Input: part model. Units: mm. Frame: model coordinates. Face numbers are marked on the shaded views. A direction names the side the tool comes from. Coordinates: 2 decimals unless noted, no trailing zeros. Loops run counter-clockwise (first coordinate to the right, second up) from the corner with the lowest first, then second, coordinate; pieces in that order, holes last. Notation, with made-up numbers: (58, 87.25) - (99, 87.25) arc R29 ccw to (99, 123.25) - close; hole circle Ø5 at (74, 24). An arc over 180 degrees is marked (long way). Write item = value, one per line. Start each with the question number.
from build123d import *

# Parameters (mm, degrees)
SKETCH_1_W          = 60
SKETCH_1_H          = 30
EXTRUDE_1_DEPTH     = 9
SKETCH_2_W          = 25
SKETCH_2_H          = 55
EXTRUDE_2_DEPTH     = 10
SKETCH_3_W          = 20
SKETCH_3_H          = 40
EXTRUDE_3_DEPTH     = 25
SKETCH_4_W          = 20
SKETCH_4_H          = 5
EXTRUDE_4_DEPTH     = 4
FILLET_1_R          = 4
FILLET_2_R          = 3
FILLET_3_R          = 3
EXTRUDE_5_DEPTH     = 4
EXTRUDE_6_DEPTH     = 4
FILLET_4_R          = 2
CHAMFER_1_SIZE      = 1
SKETCH_7_W          = 40
SKETCH_7_H          = 20
EXTRUDE_7_DEPTH     = 25
SKETCH_8_W          = 5
SKETCH_8_H          = 20
EXTRUDE_8_DEPTH     = 4
CHAMFER_2_SIZE      = 1
FILLET_6_R          = 2
SKETCH_9_R          = 3
CUT_EXTRUDE_1_DEPTH = 2


with BuildPart() as part:
    # 草图1 → 凸台-拉伸1 (new body)
    with BuildSketch(Plane.XY):
        Rectangle(SKETCH_1_W, SKETCH_1_H)
    extrude(amount=EXTRUDE_1_DEPTH)

    # 草图2 → 凸台-拉伸2 (add)
    with BuildSketch(Plane.XZ.offset(15)):
        with Locations((42.5, -3.5)):
            Rectangle(SKETCH_2_W, SKETCH_2_H)
    extrude(amount=-EXTRUDE_2_DEPTH)

    # 草图3 → 凸台-拉伸3 (add)
    with BuildSketch(Plane(origin=(0, -5, 0), x_dir=(1, 0, 0), z_dir=(0, 1, 0))):
        with Locations((42.5, 3.5)):
            Rectangle(SKETCH_3_W, SKETCH_3_H)
    extrude(amount=EXTRUDE_3_DEPTH)

    # 草图4 → 凸台-拉伸4 (add)
    with BuildSketch(Plane(origin=(0, -5, 0), x_dir=(1, 0, 0), z_dir=(0, 1, 0))):
        with Locations((42.5, 26)):
            Rectangle(SKETCH_4_W, SKETCH_4_H)
        with Locations((42.5, -19)):
            Rectangle(SKETCH_4_W, SKETCH_4_H)
    extrude(amount=EXTRUDE_4_DEPTH)

    # 圆角1
    fillet_1_edges = [part.edges().sort_by_distance(p)[0] for p in [
        (30, -10, -31),
        (30, -10, 24),
        (55, -10, 24),
        (55, -10, -31),
    ]]
    fillet(fillet_1_edges, radius=FILLET_1_R)

    # 圆角2
    fillet_2_edges = [part.edges().sort_by_distance(p)[0] for p in [
        (52.5, -3, -28.5),
        (32.5, -3, -28.5),
        (52.5, -3, 21.5),
        (32.5, -3, 21.5),
    ]]
    fillet(fillet_2_edges, radius=FILLET_2_R)

    # 圆角3
    fillet_3_edges = [part.edges().sort_by_distance(p)[0] for p in [
        (-30, -15, 4.5),
        (-30, 15, 4.5),
        (30, 15, 4.5),
    ]]
    fillet(fillet_3_edges, radius=FILLET_3_R)

    # 草图5 → 凸台-拉伸5 (add)
    with BuildSketch(Plane.XZ.offset(15)):
        with BuildLine():
            Line((34, 24), (66, 24))
            ThreePointArc((66, 24), (70, 20), (66, 16))
            Line((66, 16), (34, 16))
            ThreePointArc((34, 16), (30, 20), (34, 24))
        make_face()
        with BuildLine():
            Line((35, 10), (75, 10))
            ThreePointArc((75, 10), (80, 5), (75, 0))
            Line((75, 0), (35, 0))
            ThreePointArc((35, 0), (30, 5), (35, 10))
        make_face()
    extrude_5 = extrude(amount=EXTRUDE_5_DEPTH)

    # 镜向1: 凸台-拉伸5 across plane
    add(extrude_5.mirror(Plane(origin=(0, 0, -3.5), x_dir=(1, 0, 0), z_dir=(0, 0, -1))))

    # 草图6 → 凸台-拉伸6 (add)
    with BuildSketch(Plane(origin=(0, -15, 0), x_dir=(1, 0, 0), z_dir=(0, 1, 0))):
        Polygon((62, 34), (77, 6), (127, 6), (127, 10.5), align=None)
    extrude_6 = extrude(amount=EXTRUDE_6_DEPTH)

    # 镜向2: 凸台-拉伸6 across plane
    add(extrude_6.mirror(Plane(origin=(0, 0, -3.5), x_dir=(1, 0, 0), z_dir=(0, 0, -1))))

    # 圆角4
    # the kernel refuses this fillet: 2 mm, written as the material it takes off along each edge
    with BuildSketch(Plane(origin=(62, -15, -34), x_dir=(0.47222141251542, 0, 0.8814799700287814), z_dir=(0, 1, 0))) as fillet_4_piece_1:
        with BuildLine():
            CenterArc((FILLET_4_R * 2.60886248276, FILLET_4_R), FILLET_4_R, 131.944537695, 138.055462305)
            Line((FILLET_4_R * 1.94045155385, FILLET_4_R * 1.74379219551), (0, 0))
            Line((0, 0), (FILLET_4_R * 2.60886248276, 0))
        make_face()
    extrude(amount=17.044312414, mode=Mode.SUBTRACT)
    with BuildSketch(Plane(origin=(62, -15, 27), x_dir=(0.47222141251541977, 0, -0.8814799700287816), z_dir=(0, 1, 0))) as fillet_4_piece_2:
        with BuildLine():
            CenterArc((FILLET_4_R * 2.60886248276, -FILLET_4_R), FILLET_4_R, 90, 138.055462305)
            Line((FILLET_4_R * 1.94045155385, -FILLET_4_R * 1.74379219551), (0, 0))
            Line((0, 0), (FILLET_4_R * 2.60886248276, 0))
        make_face()
    extrude(amount=17.044312414, mode=Mode.SUBTRACT)

    # 倒角1
    chamfer_1_edges = [part.edges().sort_by_distance(p)[0] for p in [
        (32.5, 20, -3.5),
        (42.5, 20, 16.5),
        (52.5, 20, -3.5),
        (42.5, 20, -23.5),
    ]]
    chamfer(chamfer_1_edges, length=CHAMFER_1_SIZE)

    # 草图7 → 凸台-拉伸7 (add)
    with BuildSketch(Plane(origin=(0, 0, 0), x_dir=(-1, 0, 0), z_dir=(0, 0, -1))):
        Rectangle(SKETCH_7_W, SKETCH_7_H)
    extrude(amount=EXTRUDE_7_DEPTH)

    # 草图8 → 凸台-拉伸8 (add)
    with BuildSketch(Plane(origin=(0, 0, 0), x_dir=(-1, 0, 0), z_dir=(0, 0, -1))):
        with Locations((22.5, 0)):
            Rectangle(SKETCH_8_W, SKETCH_8_H)
        with Locations((-22.5, 0)):
            Rectangle(SKETCH_8_W, SKETCH_8_H)
    extrude(amount=EXTRUDE_8_DEPTH)

    # 倒角2
    chamfer_2_edges = [part.edges().sort_by_distance(p)[0] for p in [
        (-20, 0, -25),
        (0, 10, -25),
        (20, 0, -25),
        (0, -10, -25),
    ]]
    chamfer(chamfer_2_edges, length=CHAMFER_2_SIZE)

    # 圆角6
    fillet_6_edges = [part.edges().sort_by_distance(p)[0] for p in [
        (-25, -10, -2),
        (-25, 10, -2),
        (25, 10, -2),
        (25, -10, -2),
    ]]
    fillet(fillet_6_edges, radius=FILLET_6_R)

    # 草图9 → 切除-拉伸1 (cut)
    with BuildSketch(Plane.XY.offset(9)):
        with Locations((-10, 0)):
            Circle(SKETCH_9_R)
    extrude(amount=-CUT_EXTRUDE_1_DEPTH, mode=Mode.SUBTRACT)


solid = part.part
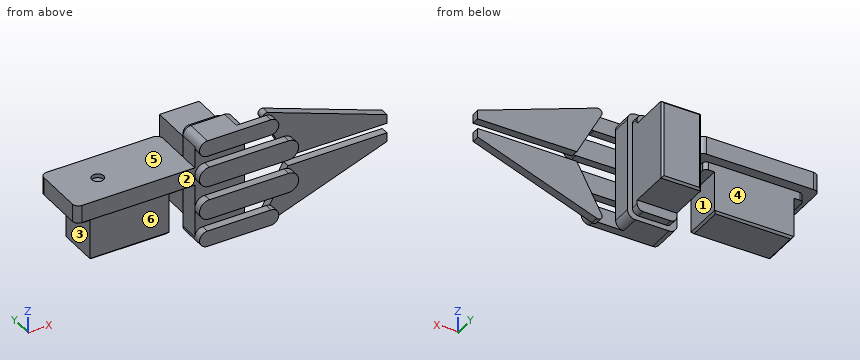
Item 1: Cut plane B-B on z = -20. Return loops of the section in (x, y).
Item 2: Pull-direction query (X, two-part tool) for the marked faces 1, 2 and 3; classes: pulls with the +X half, pulls with the -X half, needs draft (parallel to the pull), parting line crosses it, or undercut.
Item 3: Cut plane C-C on x = 98. Return loops of the section in (y, z).
Item 4: Ray query, line 1 (Z direction, x = 65.5, y = -16); line 2 (Y direction, x = -10, z = 7.7); line 3 (X direction, y = 15.5, z = -13.5). Return the intervals inside material, ascending.
Item 5: Access query for the marked faces 4, 5 and 6. Directions: +Z, -Z, +X, -X, +Y, -Y. A direction counts if a zero-diameter tool reaches every point of the face in a straight line with its end or side. Return the directions, or none.
Item 6: Cut plane A-A on x = 81.5. Return loops of the section in (y, z).
Item 7: Pin query (flat end, axial travel): pin 1 (6.5 mm diameter, centred on x = 62, z = 21, fed in from +Y); pin 2 (6 mm diameter, centred on y = -4.5, z = -16, fed in from -X); pin 3 (10 mm diameter, centred on x = 38.5, y = 8.5, fed in from -Z). Return the tip coordinate at first contact, or that it passes through.
Recorded:
q1.outline = (-20, -10) - (20, -10) - (20, 10) - (-20, 10) - close; (30, -15) - (55, -15) - (55, -5) - (52.5, -5) - (52.5, 19) - (51.5, 20) - (33.5, 20) - (32.5, 19) - (32.5, -5) - (30, -5) - close; (69.5, -15) - (100.72, -15) - (100.72, -11) - (69.5, -11) - close
q2.face_1 = undercut
q2.face_2 = needs draft
q2.face_3 = pulls with the -X half
q3.outline = (-15, -20.98) - (-11, -20.98) - (-11, -6) - (-15, -6) - close; (-15, -1) - (-11, -1) - (-11, 13.98) - (-15, 13.98) - close
q4.line_1 = -31 to -23, -17 to -7, 0 to 10, 16 to 24
q4.line_2 = -15 to -3, 3 to 15
q4.line_3 = 32.5 to 52.5
q5.face_4 = -Z, -X, +Y
q5.face_5 = +Z, -X, +Y, -Y
q5.face_6 = -Z, -X, -Y
q6.outline = (-15, -26.95) - (-11, -26.95) - (-11, -6) - (-15, -6) - close; (-15, -1) - (-11, -1) - (-11, 19.95) - (-15, 19.95) - close
q7.pin_1 = -11
q7.pin_2 = -20
q7.pin_3 = -23.5
